```python
from build123d import *

# Parameters (mm, degrees)
F0_W      = 80
F0_H      = 23.5
F1_DEPTH  = 14.5
F2_W      = 80
F2_H      = 2
F3_DEPTH  = 3.5
F4_R      = 6
F5_DEPTH  = 29.001
F6_R      = 9.25
F7_DEPTH  = 12.5
F8_R      = 5
F9_DEPTH  = 29.001
F10_W     = 80
F10_H     = 8
F11_DEPTH = 7
F12_R     = 2
F13_DEPTH = 8


with BuildPart() as f1:
    # F0 (on Front) → F1 (new body, symmetric)
    with BuildSketch(Plane.XZ):
        with Locations((0, 1.75)):
            Rectangle(F0_W, F0_H)
    extrude(amount=F1_DEPTH, both=True)

    # F2 (on face) → F3 (cut)
    with BuildSketch(Plane.XZ.offset(14.5)):
        with Locations((0, 12.5)):
            Rectangle(F2_W, F2_H)
    extrude(amount=-F3_DEPTH, mode=Mode.SUBTRACT)

    # F4 (on face) → F5 (cut, through all)
    with BuildSketch(Plane(origin=(0, 14.5, 0), x_dir=(-1, 0, 0), z_dir=(0, 1, 0))):
        Circle(F4_R)
    extrude(amount=-F5_DEPTH, mode=Mode.SUBTRACT)

    # F6 (on face) → F7 (cut)
    with BuildSketch(Plane(origin=(0, 14.5, 0), x_dir=(-1, 0, 0), z_dir=(0, 1, 0))):
        Circle(F6_R)
    extrude(amount=-F7_DEPTH, mode=Mode.SUBTRACT)

    # F8 (on face) → F9 (cut, through all)
    with BuildSketch(Plane.XZ.offset(14.5)):
        with Locations((-26, 0)):
            Circle(F8_R)
        with Locations((26, 0)):
            Circle(F8_R)
    extrude(amount=-F9_DEPTH, mode=Mode.SUBTRACT)

    # F10 (on face) → F11 (cut)
    with BuildSketch(Plane.XY.offset(13.5)):
        with Locations((0, -3)):
            Rectangle(F10_W, F10_H)
    extrude(amount=-F11_DEPTH, mode=Mode.SUBTRACT)

    # F12 (on face) → F13 (cut)
    with BuildSketch(Plane.XZ.offset(14.5)):
        with Locations((-30, 9)):
            Circle(F12_R)
        with Locations((30, 9)):
            Circle(F12_R)
    extrude(amount=-F13_DEPTH, mode=Mode.SUBTRACT)


solid = f1.part
```
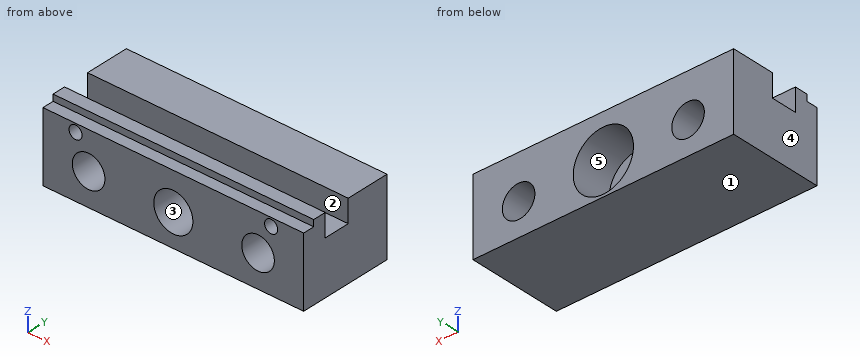
Source: CAD feature listing. Evaluate the final solid. Frame: model axes, mm. Face numbers are marked on the shaded views. A direction names the side the tool comes from. Give positions to 0.01 mm unless a question says otherwise; leave off trailing zeros. Order: outer loops, then holes, each group sorted by start corner. A loop starts at its lowest first (then second) coordinate and runs counter-clockwise, first axis right, second up.
(1) Pull-direction query (Z, two-part tool) for the marked faces 1, 2 and 3; classes: +Z half, -Z half, draft (parallel to the pull), parting line (faces both ways), or undercut.
(2) Section query B-B (x = 26). Return the cut outline in (y, z), plus the area to 4 significant figures.
(3) Access query for the marked faces 4 and 5. Directions: +Z, -Z, +X, -X, +Y, -Y. A direction counts if a zero-diameter tool reaches every point of the face in a straight line with its end or side. Return the directions, or none.
(4) Section query C-C (y = -4). Return the cut outline in (x, z), plus the area to 3 significant figures.
(5) Section query D-D (x = 0). Return the cut outline in (y, z).
(6) Material intervals for line 1 along Y through (x, z) = (-34, 6.75); line 2 along Z through (x, y) = (-30, -8.5); line 3 along X through (y, z) = (-12.75, -2), sorted ascending.
(7) Section query A-A (z = 0). Return the cut outline in (x, y).
(8) Contact query for flat-ended pins moving along their axis: P1, Ø7.5, axis at x = 0.5, z = 9, coming from the +Y side; P2, Ø6.5, axis at x = -20, y = -3, coming from the +Z side. Output: stop coordinate, or through.
Outcome:
1. face 1: -Z half
1. face 2: draft
1. face 3: undercut
2. outline: (-14.5, -10) - (14.5, -10) - (14.5, -5) - (-14.5, -5) - close; (-14.5, 5) - (14.5, 5) - (14.5, 13.5) - (1, 13.5) - (1, 6.5) - (-7, 6.5) - (-7, 13.5) - (-11, 13.5) - (-11, 11.5) - (-14.5, 11.5) - close
2. area: 328.5 mm2
3. face 4: +Z, -Z, -X, +Y, -Y
3. face 5: +Y
4. outline: (-40, -10) - (40, -10) - (40, 6.5) - (-40, 6.5) - close; hole circle Ø10 at (-26, 0); hole circle Ø12 at (0, 0); hole circle Ø10 at (26, 0)
4. area: 1,050 mm2
5. outline: (-14.5, -10) - (14.5, -10) - (14.5, -9.25) - (2, -9.25) - (2, -6) - (-14.5, -6) - close; (-14.5, 6) - (2, 6) - (2, 9.25) - (14.5, 9.25) - (14.5, 13.5) - (1, 13.5) - (1, 6.5) - (-7, 6.5) - (-7, 13.5) - (-11, 13.5) - (-11, 11.5) - (-14.5, 11.5) - close
6. line 1: y = -14.5 to -7, 1 to 14.5
6. line 2: z = -10 to -3, 3 to 7, 11 to 13.5
6. line 3: x = -40 to -30.58, -21.42 to -5.66, 5.66 to 21.42, 30.58 to 40
7. outline: (-40, -14.5) - (-31, -14.5) - (-31, 14.5) - (-40, 14.5) - close; (-21, -14.5) - (-6, -14.5) - (-6, 2) - (-9.25, 2) - (-9.25, 14.5) - (-21, 14.5) - close; (6, -14.5) - (21, -14.5) - (21, 14.5) - (9.25, 14.5) - (9.25, 2) - (6, 2) - close; (31, -14.5) - (40, -14.5) - (40, 14.5) - (31, 14.5) - close
8. P1: stops at y = 14.5
8. P2: stops at z = 6.5
